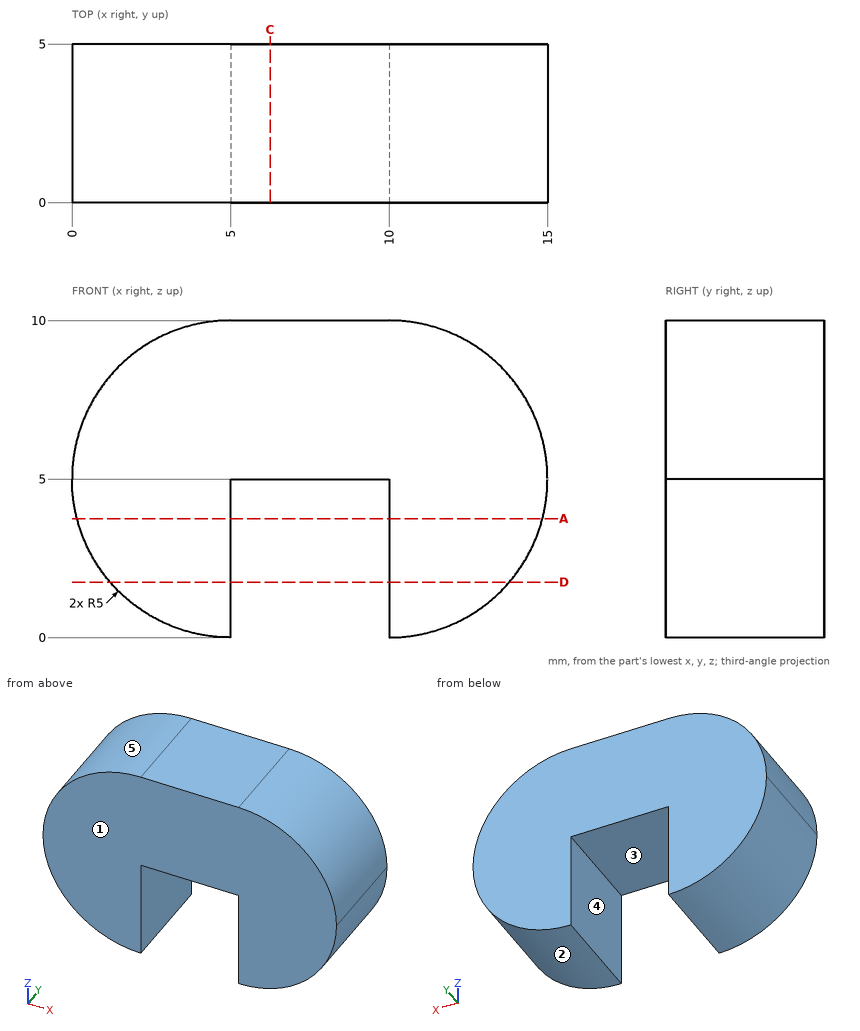
Answer from the drawing. Dimensions are ordinates in mm from the lowest x, y and z of the part. A direction names the side the tool comes from. Give positions to 0.01 mm unless a question says otherwise; leave off trailing zeros. Order: outer loops, then holes, each group sorted by start corner. A loop starts at its lowest first (then second) coordinate and runs counter-clockwise, first axis right, second up.
(1) Find section D-D (z = 1.75). Give the vertices of the cut face in (x, y).
(2) Straight lines are drawn through the part: L1, parallel to X at y = 3.35, z = 1.25; L2, parallel to Z at x = 8.5, y = 4.2; L3, parallel to X at y = 4, z = 4.75. For each, find the intervals that lie inside material, in ascending order.
(3) Given pin 1 (6 mm diameter, centred on x = 6, z = 3, fed in from -Y); pin 2 (2 mm diameter, centred on y = 2, z = 9, fed in from -X), each flat-ended and moving along its own axis, determine where each tip first touches the part or whether it passes through.
(4) For a pull along X with two mould halves and no side action, classify the marked faces 1, 2 and 3 as released by +X, released by -X, zero draft, split by the parting line, or undercut.
(5) For the marked faces 4 and 5, determine the directions among +Z, -Z, +X, -X, +Y, -Y from which every point of the face is accessible in a straight line to the end or side of a thin tool.
(6) Find section C-C (x = 6.25). Give the vertices of the cut face in (y, z).
(7) Find section A-A (z = 3.75). Give the vertices of the cut face in (x, y), plus the area to 3 significant figures.
Result sheet:
1. outline: (1.2, 0) - (5, 0) - (5, 5) - (1.2, 5) - close; (10, 0) - (13.8, 0) - (13.8, 5) - (10, 5) - close
2. L1: x = 1.69 to 5, 10 to 13.31
2. L2: z = 5 to 10
2. L3: x = 0.01 to 5, 10 to 14.99
3. pin 1: stops at y = 0
3. pin 2: stops at x = 1
4. face 1: zero draft
4. face 2: released by +X
4. face 3: undercut
5. face 4: -Z, +Y, -Y
5. face 5: +Z, -X, +Y, -Y
6. outline: (0, 5) - (5, 5) - (5, 10) - (0, 10) - close
7. outline: (0.16, 0) - (5, 0) - (5, 5) - (0.16, 5) - close; (10, 0) - (14.84, 0) - (14.84, 5) - (10, 5) - close
7. area: 48.4 mm2
